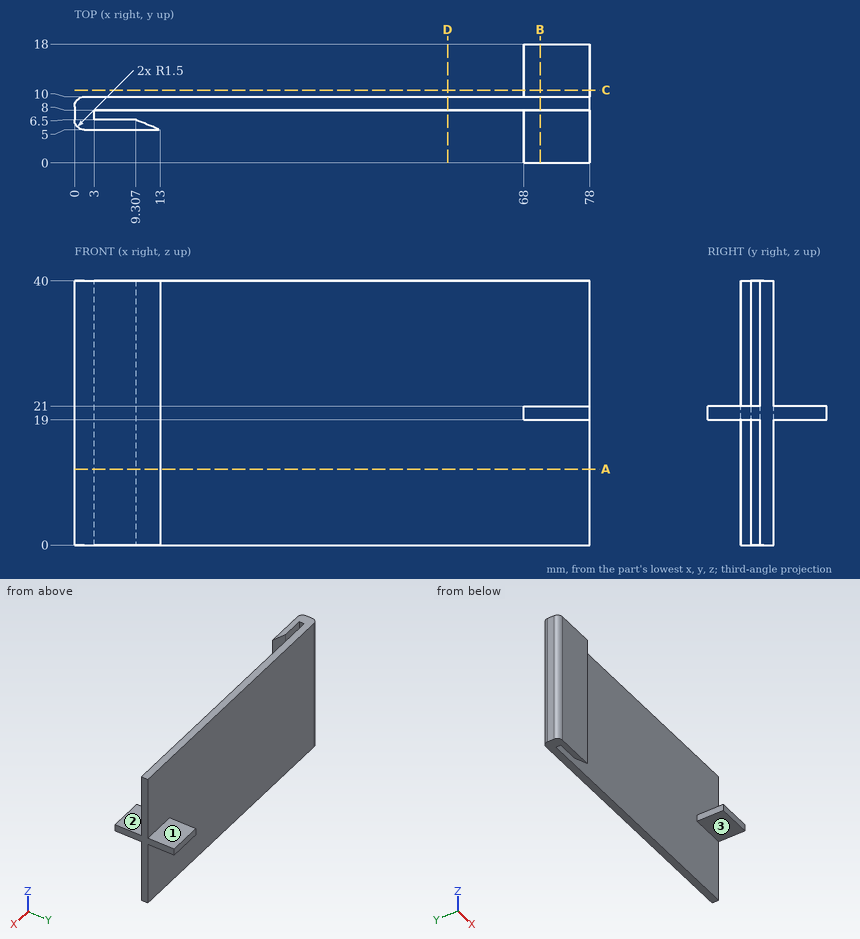
Part print with two shaded views. Sizes in mm from the minimum x, y, z corner. A direction names the side the tool comes from. Give positions to 0.01 mm unless a question says otherwise; leave off trailing zeros. Order: outer loops, then holes, each group sorted by start corner. A loop starts at its lowest first (then second) coordinate and runs counter-clockwise, first axis right, second up.
1) Wall check: probe 1 along Y at (x, z) = (72, 5.5); probe 2 along Y at (x, z) = (12.5, 34); probe 3 along Z at (x, y) = (71.5, 15). Give the ranges that are in metal, low to high.
2) Saw through at A-A, the plane z = 11.5. Write the cut outline in (x, y), then the cut area to 3 significant figures.
3) 3-axis set-ups, long thin cutter, end or side, ignore diameter. For the marked faces 1, 2 and 3: which of +Z, -Z, +X, -X, +Y, -Y reach the whole face in a straight line?
4) Saw through at C-C, the plane y = 11. Write the cut outline in (x, z), then the cut area to 3 significant figures.
5) Saw through at B-B, the plane x = 70.5. Write the cut outline in (y, z).
6) Pin check, flat tips, straight feed: pin 1 (9 mm diameter, centred on x = 73, y = 13, fed in from -Z); pin 2 (1.6 mm diameter, centred on y = 12, z = 20, fed in from -X); pin 3 (1 mm diameter, centred on x = 28.5, z = 19, fed in from -Y); pin 4 (1.9 mm diameter, centred on x = 7.5, z = 26, fed in from +Y). Stop position of each tip, or through.
7) Saw through at D-D, the plane x = 56.5. Write the cut outline in (y, z).
Computed:
1. probe 1: y = 8 to 10
1. probe 2: y = 5 to 5.2, 8 to 10
1. probe 3: z = 19 to 21
2. outline: (0, 6.5) arc R1.5 ccw to (1.5, 5) - (13, 5) - (9.31, 6.5) - (3, 6.5) - (3, 8) - (78, 8) - (78, 10) - (1.5, 10) arc R1.5 ccw to (0, 8.5) - close
2. area: 176 mm2
3. face 1: +Z, +X, -X, +Y
3. face 2: +Z, +X, -Y
3. face 3: -Z, +X, -Y
4. outline: (68, 19) - (78, 19) - (78, 21) - (68, 21) - close
4. area: 20.0 mm2
5. outline: (0, 19) - (8, 19) - (8, 0) - (10, 0) - (10, 19) - (18, 19) - (18, 21) - (10, 21) - (10, 40) - (8, 40) - (8, 21) - (0, 21) - close
6. pin 1: stops at z = 0
6. pin 2: stops at x = 68
6. pin 3: stops at y = 8
6. pin 4: stops at y = 10
7. outline: (8, 0) - (10, 0) - (10, 40) - (8, 40) - close
